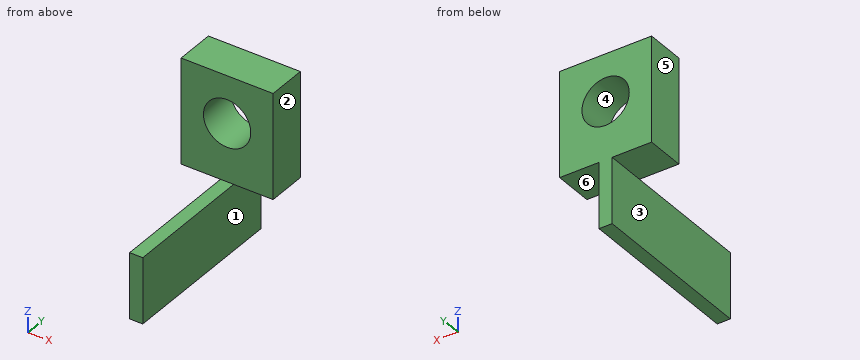
```python
from build123d import *

# Parameters (mm, degrees)
BOSS_EXTRUDE1_DEPTH  = 0.5
SKETCH2_W            = 7
SKETCH2_H            = 8
BOSS_EXTRUDE2_DEPTH  = 3
M3_CLEARANCE_HOLE1_D = 3.6


with BuildPart() as part:
    # Sketch1 → Boss-Extrude1 (new body, symmetric)
    with BuildSketch(Plane(origin=(0, 0, 0), x_dir=(0, 0, -1), z_dir=(1, 0, 0))):
        Polygon((0, 0), (0, 10), (-8, 10), (-8, 13), (5, 13), (5, 0), align=None)
    extrude(amount=BOSS_EXTRUDE1_DEPTH, both=True)

    # Sketch2 → Boss-Extrude2 (add, through all)
    with BuildSketch(Plane.XZ.offset(-10)):
        with Locations((0, 4)):
            Rectangle(SKETCH2_W, SKETCH2_H)
    extrude(amount=-BOSS_EXTRUDE2_DEPTH)

    # M3 Clearance Hole1 (through all)
    with Locations(Plane(origin=(0, 13, 0), x_dir=(1, 0, 0), z_dir=(0, 1, 0))):
        with Locations((0, -4.401597527)):
            Hole(M3_CLEARANCE_HOLE1_D / 2)


solid = part.part
```
Work out the finished part from the listing and answer in its coordinate system (mm). Face numbers are marked on the shaded views. A direction names the side the tool comes from. Give positions to 0.01 mm unless a question says otherwise; leave off trailing zeros. Loops run counter-clockwise (first coordinate to the right, second up) from the corner with the lowest first, then second, coordinate; pieces in that order, holes last. Notation, with made-up numbers: (46, 10) -> (70, 10) arc R36 cw to (70, 48) -> close; hole circle Ø8 at (-13, -38). An arc over 180 degrees is marked (long way). One line per question, with ' | ' between items. Start each with the question number.
1) For the marked faces 1, 2 and 3, determine the directions among +Z, -Z, +X, -X, +Y, -Y from which every point of the face is accessible in a straight line to the end or side of a thin tool.
2) Section C-C, the plane y = 11 is taken. Determine the outline of the cut face in (x, z).
3) Determine the mould class of the marked faces 4, 5 and 6 for opening direction X: +X half, -X half, draft (parallel to the pull), parting line (faces both ways), or undercut.
4) Straight lines are drawn through the part: L1, parallel to Z at x = 0, y = 11.3; L2, parallel to X at y = 11, z = -0.5; L3, parallel to Y at x = -3, z = 6.25. For each, find the intervals that lie inside material, in ascending order.
5) Section D-D, the plane x = 1.5 is taken. Determine the outline of the cut face in (y, z).
6) Each of these flat-tipped pins is pushed along its axis until it touches: pin 1 (3.5 mm diameter, centred on x = 1.5, y = 12, fed in from -Z); pin 2 (2.5 mm diameter, centred on y = 3.5, z = -2, fed in from -X); pin 3 (4 mm diameter, centred on x = 1.5, y = 6, fed in from +Z); pin 4 (1.5 mm diameter, centred on y = 9, z = -2.5, fed in from +X). Where does it stop, or does it pass through?
7) Section B-B, the plane z = 5 is taken. Determine the outline of the cut face in (x, y), then the cut area to 3 significant figures.
8) Section A-A, the plane x = 0 is taken. Determine the outline of the cut face in (y, z), then the cut area to 3 significant figures.
Resolved:
1) face 1: -Z, +X, +Y, -Y | face 2: +Z, -Z, +X, +Y, -Y | face 3: -Z, -X, +Y, -Y
2) outline: (-3.5, 0) -> (-0.5, 0) -> (-0.5, -5) -> (0.5, -5) -> (0.5, 0) -> (3.5, 0) -> (3.5, 8) -> (-3.5, 8) -> close; hole circle Ø3.6 at (0, 4.4)
3) face 4: undercut | face 5: -X half | face 6: draft
4) L1: -5 to 2.6, 6.2 to 8 | L2: -0.5 to 0.5 | L3: 10 to 13
5) outline: (10, 0) -> (13, 0) -> (13, 3.41) -> (10, 3.41) -> close; (10, 5.4) -> (13, 5.4) -> (13, 8) -> (10, 8) -> close
6) pin 1: z = -5 | pin 2: x = -0.5 | pin 3: z = 0 | pin 4: x = 0.5
7) outline: (-3.5, 10) -> (-1.7, 10) -> (-1.7, 13) -> (-3.5, 13) -> close; (1.7, 10) -> (3.5, 10) -> (3.5, 13) -> (1.7, 13) -> close | area: 10.8 mm2
8) outline: (0, -5) -> (13, -5) -> (13, 2.6) -> (10, 2.6) -> (10, 0) -> (0, 0) -> close; (10, 6.2) -> (13, 6.2) -> (13, 8) -> (10, 8) -> close | area: 78.2 mm2
